CAD build for the part. Positions are in the model's coordinates, mm. Give positions to 0.01 mm unless a question says otherwise; leave off trailing zeros. Write each loop counter-clockwise with the first axis right and the second up, starting at its lowest first coordinate (ties: lowest second). Pieces come first, ordered by that corner, then holes. Notation, with made-up numbers: M 31.25,64.5 L 39.25,64.5 A30 cw 39.25,103.5 Z; hole C 22,68 d11. An arc over 180 degrees is marked long. One line per question, with ' | ' between items. Start each with the question number.
1. Cut at A-A, the plane y = 0. Write the cut outline in (x, z).
2. Cut at B-B, the plane x = -12. Write the cut outline in (y, z), then the cut area to 3 significant figures.
3. Pull direction X, two halves, no side cores. Call faces 1 (the face through (0, -34, 5)), 2 (the face through (-31.22, -1.37, 4.93)), 3 (the face through (-2, 37, 4)): released by +X, released by -X, zero draft, split by the parting line, or undercut.
4. Cut at C-C, the plane z = 7.5. Count the separate pieces of the cut face and the enclosed holes in it, then the cut area to 3 significant figures.
5. Wall check: L1, parallel to Y at x = 0, z = 6.75; L2, parallel to Y at x = 0, z = 4.5; L3, parallel to Y at x = 0, z = 2. Give the ranges that are in metal, low to high.
6. Flat gauge pins, fed straight in: pin 1 (3.5 mm diameter, centred on x = 0, y = 35, fed in from -Z); pin 2 (2 mm diameter, centred on y = 27, z = 4, fed in from +X); pin 3 (1.5 mm diameter, centred on y = 25, z = 1.5, fed in from -X); pin 4 (2 mm diameter, centred on y = -10, z = 6.5, fed in from +X). Where does each tip first touch, or does it go through?
Autodesk Fusion 360 part; units mm, degrees
sketch "Sketch2" plane through (0, 0, 0) normal (0, 0, 1) x (1, 0, 0)
  circle A0 centre (0, 0) radius 34
  circle A1 centre (0, 0) radius 22.5
  circle A2 centre (0, 0) radius 31.25
  line L0 (0, 0) -> (0, 35) construction
  circle A3 centre (0, 35) radius 2.15
  circle A4 centre (0, 35) radius 4.15
  circle A5 centre (-30.3109, -17.5) radius 4.15
  circle A6 centre (-30.3109, -17.5) radius 2.15
  circle A7 centre (30.3109, -17.5) radius 4.15
  circle A8 centre (30.3109, -17.5) radius 2.15
  dimension "d19" = 68
  dimension "d21" = 45
  dimension "d29" = 62.5
  dimension "d75" = 35
  dimension "d76" = 4.3
  dimension "d78" = 2
  dimension "d80" = 360
extrude "main" add sketch "Sketch2" along normal blind 10 contours A0 A2 A4 A7 | A0 A2 A3 A4 | A0 A3 A4 | A0 A7 A8 | A0 A2 A7 A8 | A0 A2 A4 A5 | A0 A2 A5 A7 | A0 A2 A5 A6 | A0 A5 A6
chamfer "Chamfer4" distance 5 angle 45 6 edges at (31.2257, -13.4521, 5) (3.963, 33.7683, 5) (-3.963, 33.7683, 5) (-31.2257, -13.4521, 5) (-27.2627, -20.3162, 5) (27.2627, -20.3162, 5)
sketch "Sketch4" plane through (0, 0, 0) normal (1, 0, 0) x (0, 1, 0)
  line L0 (0, 0) -> (33, 0) construction
  line L1 (33, 0) -> (49.4315, 16.4315)
  line L2 (33, 0) -> (56.2377, 0)
  line L3 (49.4315, 16.4315) -> (49.4315, 0)
  dimension "d69" = 33
  dimension "d70" = 45
extrude "Extrude8" cut sketch "Sketch4" along normal mid plane 20
pattern_circular "C-Pattern3" count 3 over 360 about axis through (0, 0, 1.75) along (0, 0, 1) of "Extrude8"
equation "gear_OD = ( gear_Nr * diameter_scale * module ) + 8 mm"
equation "ring_width = 52 mm"
equation "m3_hole_thickness = 2 mm"
equation "m3_inserts = 4.3 mm"
equation "d19 = gear_OD"
equation "output_bearing_od = 47 mm"
equation "d21 = output_bearing_od - 2 mm"
equation "d29 = gear_OD - wall_thickness + 1.5 mm"
equation "wall_thickness = 7 mm"
equation "d33 = height"
equation "height = 10 mm"
equation "helix_angle = 0 deg"
equation "diameter_scale = ( 1 / cos(helix_angle) ) * 1 mm"
equation "d69 = ( gear_OD / 2 ) - 1 mm"
equation "d75 = ( gear_OD / 2 ) + 1 mm"
equation "d76 = m3_inserts"
equation "d78 = m3_hole_thickness"
Here are the results:
1) outline: M -34,0 L -31.25,0 L -31.25,10 L -34,10 Z; M 31.25,0 L 34,0 L 34,10 L 31.25,10 Z
2) outline: M -31.81,0 L -28.85,0 L -28.85,10 L -31.81,10 Z; M 28.85,0 L 31.81,0 L 31.81,10 L 28.85,10 Z | area: 59.2 mm^2
3) face 1: split by the parting line | face 2: undercut | face 3: zero draft
4) separate pieces: 1 | enclosed holes: 4 | area: 673 mm^2
5) L1: -34 to -31.25, 31.25 to 32.85, 37.15 to 39.15 | L2: -34 to -31.25, 31.25 to 32.85, 37.15 to 37.5 | L3: -34 to -31.25, 31.25 to 32.85
6) pin 1: through | pin 2: x = 21.91 | pin 3: x = -23.83 | pin 4: x = 33.28
